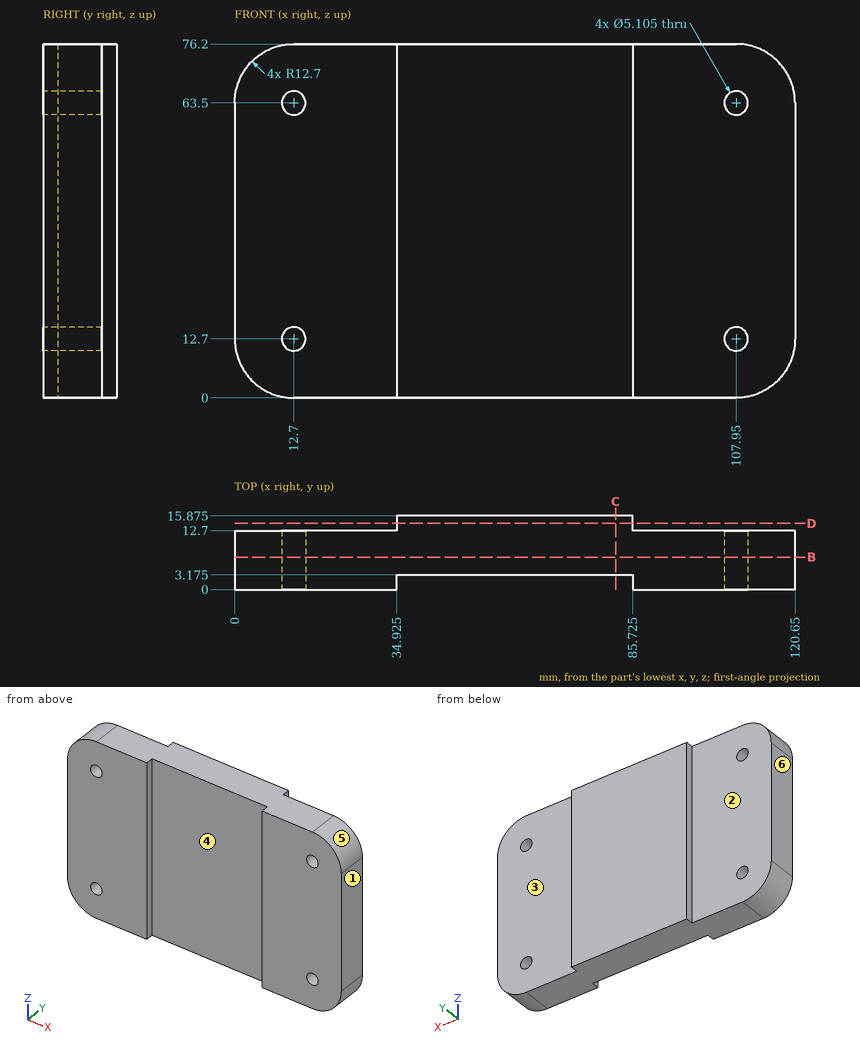
Could you check a few things on this drawing? It's one solid part, dimensions in mm from its lowest x, y, z. A direction names the side the tool comes from. Round coordinates to 2 decimals unless told otherwise and drop trailing zeros. Write each loop counter-clockwise with the first axis right and the second up, starting at its lowest first coordinate (ties: lowest second). Pieces come first, ordered by that corner, then holes. Notation, with made-up numbers: M 70,13 L 79,13 A17 ccw 79,42 Z; hole C 83,22 d1. An arc over 180 degrees is marked long. Answer as CSV lines item,"result". Start each with the question number.
1. On a 3-axis mill with a long thin cutter (end or side, diameter ignored), from which of +Z, -Z, +X, -X, +Y, -Y can I reach the whole of each face in a straight line? I mean the marked faces 1, 2 and 3. Say none if no direction works.
2. I'm going to push flat-ended pins straight in: pin 1 Ø4 at (x, z) = (12.7, 12.7) entering from -Y; pin 2 Ø15 at (x, z) = (62, 38.5) entering from -Y (3 decimals); pin 3 Ø1.5 at (x, z) = (21, 17) entering from +Y; pin 4 Ø2.5 at (y, z) = (14.5, 51) entering from +X (3 decimals). Where does each tip first touch, or does it pass through?
3. I need wall thicknesses on probe 1 along Z at (x, y) = (107.95, 10.25); probe 2 along Z at (x, y) = (12, 12.5) (1 decimal); probe 3 along Y at (x, z) = (28.5, 70.5). Which ranges of each line are inside material? Lowest first, please.
4. Suppose I cut it at D-D on y = 14.25. Write out the boundary of the cut face in (x, z) (1 decimal).
5. Suppose I cut it at B-B on y = 7. Count the separate pieces of the cut face and the enclosed holes in it, then the cut area to 3 significant figures.
6. Suppose I cut it at C-C on x = 82. Write out the boundary of the cut face in (y, z) (1 decimal).
7. Thinking about a two-plate mould opening in X: for the marked faces 4, 5 and 6, which applies, released by +X, released by -X, zero draft, split by the parting line, or undercut?
Check result:
1,face 1,"+Z, -Z, +X, +Y, -Y"
1,face 2,"+Z, -Z, -X, +Y"
1,face 3,"+Z, -Z, +X, +Y"
2,pin 1,"passes through"
2,pin 2,"stops at y = 3.175"
2,pin 3,"stops at y = 12.7"
2,pin 4,"stops at x = 85.725"
3,probe 1,"z = 0 to 10.15, 15.25 to 60.95, 66.05 to 76.2"
3,probe 2,"z = 0 to 10.2, 15.2 to 61, 66 to 76.2"
3,probe 3,"y = 0 to 12.7"
4,outline,"M 34.9,0 L 85.7,0 L 85.7,76.2 L 34.9,76.2 Z"
5,separate pieces,"1"
5,enclosed holes,"4"
5,area,"8,970 mm2"
6,outline,"M 3.2,0 L 15.9,0 L 15.9,76.2 L 3.2,76.2 Z"
7,face 4,"undercut"
7,face 5,"released by +X"
7,face 6,"released by -X"
